from build123d import *

# Parameters (mm, degrees)
SKETCH1_W           = 25.4
SKETCH1_H           = 50.8
BOSS_EXTRUDE1_DEPTH = 6.35
CUT_EXTRUDE1_DEPTH  = 30.099355663
CUT_EXTRUDE2_DEPTH  = 30.099355663


with BuildPart() as part:
    # Sketch1 → Boss-Extrude1 (new body)
    with BuildSketch(Plane.XY):
        Rectangle(SKETCH1_W, SKETCH1_H)
    extrude(amount=BOSS_EXTRUDE1_DEPTH)

    # Sketch2 → Cut-Extrude1 (cut, through all)
    with BuildSketch(Plane.XY.offset(6.35)):
        with BuildLine():
            Line((-1.5875, 22.023361062), (-1.5875, 14.440204949))
            Line((-1.5875, 14.440204949), (1.5875, 14.440204949))
            Line((1.5875, 14.440204949), (1.5875, 22.023361062))
            ThreePointArc((1.5875, 22.023361062), (0, 22.225), (-1.5875, 22.023361062))
        make_face()
        with BuildLine():
            Line((1.5875, 14.440204949), (-1.5875, 14.440204949))
            Line((-1.5875, 14.440204949), (-1.5875, 22.023361062))
            ThreePointArc((-1.5875, 22.023361062), (-3.888564967, 10.854884214), (6.35, 15.875))
            ThreePointArc((6.35, 15.875), (5.020115786, 19.763564967), (1.5875, 22.023361062))
            Line((1.5875, 22.023361062), (1.5875, 14.440204949))
        make_face()
        with BuildLine():
            Line((-1.5875, 25.4), (-1.5875, 22.023361062))
            ThreePointArc((-1.5875, 22.023361062), (0, 22.225), (1.5875, 22.023361062))
            Line((1.5875, 22.023361062), (1.5875, 25.4))
            Line((1.5875, 25.4), (-1.5875, 25.4))
        make_face()
    extrude(amount=-CUT_EXTRUDE1_DEPTH, mode=Mode.SUBTRACT)

    # Sketch3 → Cut-Extrude2 (cut, through all)
    with BuildSketch(Plane.XY.offset(6.35)):
        with BuildLine():
            Line((-3.175, -19.05), (-3.175, 0))
            ThreePointArc((-3.175, 0), (0, 3.175), (3.175, 0))
            Line((3.175, 0), (3.175, -19.05))
            ThreePointArc((3.175, -19.05), (0, -22.225), (-3.175, -19.05))
        make_face()
    extrude(amount=-CUT_EXTRUDE2_DEPTH, mode=Mode.SUBTRACT)


solid = part.part
The listing builds one solid part. Answer for the finished solid, in the listing's coordinates (mm). A direction names the side the tool comes from. Coordinates: 2 decimals unless noted, no trailing zeros. Write each loop counter-clockwise with the first axis right and the second up, starting at its lowest first coordinate (ties: lowest second). Pieces come first, ordered by that corner, then holes. Notation, with made-up numbers: M 81.5,-34.75 L 95.5,-34.75 A17 ccw 95.5,-14.75 Z; hole C 37,33 d2. An arc over 180 degrees is marked long. Put each result on its own line as item: value. Start each with the question number.
1. For a pull along Y with two mould halves and no side action, classify faces 1 (the flat face through (0, -25.4, 3)), 2 (the cylindrical face through (-0.07, 3.174, 3.219)), 3 (the flat face through (12.7, 0, 3)), 4 (the flat face through (7, 25.4, 3)) as pulls with the +Y half, pulls with the -Y half, needs draft (parallel to the pull), parting line crosses it, or undercut.
2. A flat-ended cylindrical pin translates along its axis: P1, Ø6, axis at x = -2, y = -8.5, coming from the +Z side. Find the tip coordinate at first contact, or state that the pin passes through.
3. A cutting plane is placed at B-B on x = 0. Write down the section's boundary in (y, z) (3 decimals), then the cut area to 3 significant figures.
4. A cutting plane is placed at A-A on y = -5.5. Write down the section's boundary in (x, z) (3 decimals), then the cut area to 3 significant figures.
5. Which of the six approach directions +Z, -Z, +X, -X, +Y, -Y give full straight-line access (tool end or side, diameter ignored) to faces 5 (the flat face through (-3.175, -10, 3)), 6 (the flat face through (-7, 25.4, 3)), 7 (the flat face through (1.588, 24, 3))?
6. Consider line 1 (Y direction, x = 0, z = 4.5) (3 decimals); line 2 (X direction, y = -4, z = 6) (3 decimals); line 3 (X direction, y = 19.5, z = 5.5). Determine where each line is inside the solid, lowest interval first. Write a range as from..to.
Resolved:
1. face 1: pulls with the -Y half
1. face 2: undercut
1. face 3: needs draft
1. face 4: pulls with the +Y half
2. P1: stops at z = 6.35
3. outline: M -25.4,0 L -22.225,0 L -22.225,6.35 L -25.4,6.35 Z; M 3.175,0 L 9.525,0 L 9.525,6.35 L 3.175,6.35 Z
3. area: 60.5 mm2
4. outline: M -12.7,0 L -3.175,0 L -3.175,6.35 L -12.7,6.35 Z; M 3.175,0 L 12.7,0 L 12.7,6.35 L 3.175,6.35 Z
4. area: 121 mm2
5. face 5: +Z, -Z
5. face 6: +Z, -Z, +X, -X, +Y
5. face 7: +Z, -Z, +Y
6. line 1: y = -25.4..-22.225, 3.175..9.525
6. line 2: x = -12.7..-3.175, 3.175..12.7
6. line 3: x = -12.7..-5.21, 5.21..12.7
